CAD build for the part. Positions are in the model's coordinates, mm. Face numbers are marked on the shaded views. A direction names the side the tool comes from. Give positions to 0.01 mm unless a question says otherwise; leave off trailing zeros. Order: outer loops, then holes, each group sorted by start corner. A loop starts at its lowest first (then second) coordinate and runs counter-clockwise, first axis right, second up. Notation, with made-up numbers: M 13,85.5 L 19,85.5 A20 cw 19,119.5 Z; hole C -34,14 d6. An arc over 180 degrees is marked long. Put each result on its own line as item: value. Start each with the question number.
1) Cut at B-B (z = -2.15). Give the number of separate pieces and of enclosed holes in the cut face, and give its area (3 significant figures).
2) Two-plate mould, pull along X, no slides. Class the marked faces 3, 4, 5 and 6: released by +X, released by -X, zero draft, split by the parting line, or undercut.
3) Pin check, flat tips, straight feed: pin 1 (0.8 mm diameter, centred on x = -10, z = 2, fed in from +Y); pin 2 (0.8 mm diameter, centred on y = 6, z = -2, fed in from +X). Stop position of each tip, or through.
4) Cut at A-A (z = 2). Write the cut outline in (x, y), and give its area (3 significant figures).
5) Drill centre lines: line 1 (X direction, y = 4, z = 2.1); line 2 (Z direction, x = -22.5, y = 4.5); line 3 (Z direction, x = -3, y = 7.75). Where is each one in solid material? Low to high. Write a range as [from, to].
6) Tool access for the marked faces 1 and 2: list every direction of +Z, -Z, +X, -X, +Y, -Y with a clear straight run to the whole face (end or side of a thin tool).
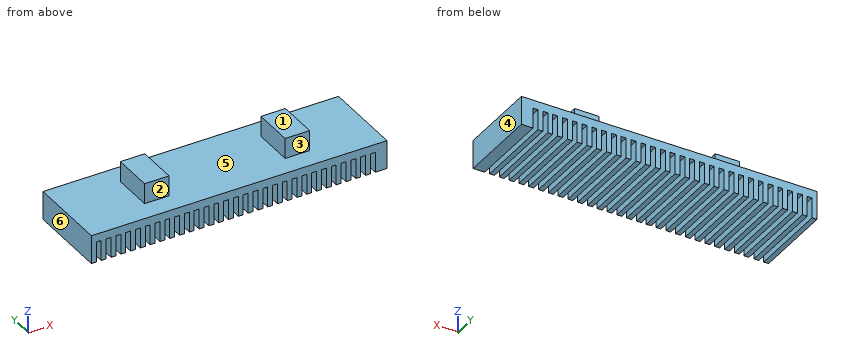
```python
from build123d import *

# Parameters (mm, degrees)
SKETCH1_W           = 36.23
SKETCH1_H           = 3.5
BOSS_EXTRUDE1_DEPTH = 10
SKETCH3_W           = 3
SKETCH3_H           = 5
BOSS_EXTRUDE2_DEPTH = 2.5
SKETCH4_W           = 0.6
SKETCH4_H           = 2.5
CUT_EXTRUDE1_DEPTH  = 11
LPATTERN1_COUNT     = 29
LPATTERN1_PITCH     = 1.2


with BuildPart() as part:
    # Sketch1 → Boss-Extrude1 (new body)
    with BuildSketch(Plane(origin=(0, 0, 0), x_dir=(1, 0, 0), z_dir=(0, 1, 0))):
        with Locations((-18.115, 1.75)):
            Rectangle(SKETCH1_W, SKETCH1_H)
    extrude(amount=BOSS_EXTRUDE1_DEPTH)

    # Sketch3 → Boss-Extrude2 (add)
    with BuildSketch(Plane.XY):
        with Locations((-26.73, 5)):
            Rectangle(SKETCH3_W, SKETCH3_H)
        with Locations((-9.5, 5)):
            Rectangle(SKETCH3_W, SKETCH3_H)
    extrude(amount=BOSS_EXTRUDE2_DEPTH)

    # Sketch4 → Cut-Extrude1 (cut, through all)
    with BuildSketch(Plane(origin=(0, 10, 0), x_dir=(1, 0, 0), z_dir=(0, 1, 0))):
        with Locations((-35.33, 2.25)):
            Rectangle(SKETCH4_W, SKETCH4_H)
    cut_extrude1 = extrude(amount=-CUT_EXTRUDE1_DEPTH, mode=Mode.SUBTRACT)

    # LPattern1: Cut-Extrude1 ×29
    with Locations(*[(i * LPATTERN1_PITCH, 0, 0) for i in range(1, LPATTERN1_COUNT)]):
        add(cut_extrude1, mode=Mode.SUBTRACT)


solid = part.part
```
Solution:
1. separate pieces: 30
1. enclosed holes: 0
1. area: 188 mm²
2. face 3: zero draft
2. face 4: released by +X
2. face 5: undercut
2. face 6: released by -X
3. pin 1: y = 7.5
3. pin 2: x = 0
4. outline: M -28.23,2.5 L -25.23,2.5 L -25.23,7.5 L -28.23,7.5 Z; M -11,2.5 L -8,2.5 L -8,7.5 L -11,7.5 Z
4. area: 30.0 mm²
5. line 1: [-28.23, -25.23], [-11, -8]
5. line 2: [-3.5, 0]
5. line 3: [-1, 0]
6. face 1: +Z, +X, -X, +Y, -Y
6. face 2: +Z, +X, -X, -Y
